from build123d import *

# Parameters (mm, degrees)
EXTRUDE_1_DEPTH = 10
FILLET_1_R      = 1


with BuildPart() as part:
    # 草图4 → 凸台-拉伸1 (new body)
    with BuildSketch(Plane.XY):
        Polygon((-29, 35), (-35, 35), (-35, 2), (-29, 2), (-29, -20), (-35, -20), (-35, -35), (35, -35), (35, 35), (29, 35), (29, 34), (17, 34), (17, 35), (-17, 35), (-17, 34), (-29, 34), align=None)
    extrude(amount=EXTRUDE_1_DEPTH)

    # 圆角1
    fillet_1_edges = [part.edges().sort_by_distance(p)[0] for p in [
        (-29, -20, 5),
        (-29, 2, 5),
        (29, 34, 5),
        (17, 34, 5),
        (-17, 34, 5),
        (-29, 34, 5),
    ]]
    fillet(fillet_1_edges, radius=FILLET_1_R - 0.0001)  # a hair under: the kernel refuses the full size


solid = part.part
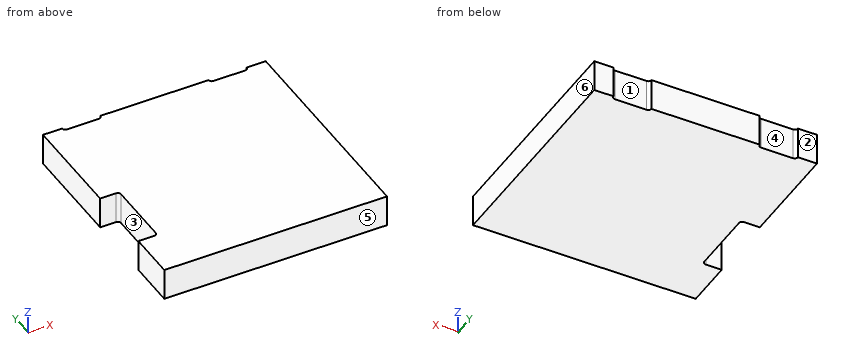
Verification items for the finished model (mm, model axes). Face numbers are marked on the shaded views. A direction names the side the tool comes from. Coordinates: 2 decimals unless noted, no trailing zeros. Order: outer loops, then holes, each group sorted by start corner. A loop starts at its lowest first (then second) coordinate and runs counter-clockwise, first axis right, second up. Notation, with made-up numbers: (-21, 6) -> (38, 6) arc R23 cw to (38, 21) -> close; hole circle Ø3 at (-2.75, 68.25). An arc over 180 degrees is marked (long way). Use CSV: the item, a comma, the result in double quotes. Start each with the question number.
Q1. Tool access check on the marked faces 1, 2 and 3. Record the directions out of +Z, -Z, +X, -X, +Y, -Y that give a thin tool (end or side, any length) a straight path to the whole face; none if there is none.
Q2. Section check B-B, the plane y = -7. Record the cut outline in (x, z).
Q3. Draft check along X on the marked faces 4, 5 and 6. Enter one of: +X half, -X half, draft (parallel to the pull), parting line (faces both ways), or undercut.
Q4. Thickness scan on line 1 along Y through (x, z) = (-31.5, 4.5); line 2 along X through (y, z) = (-11, 8.75); line 3 along Y through (x, z) = (-22, 2.5). Record the ranges inside material, lowest first.
Returned:
1,face 1,"+Z, -Z, +Y"
1,face 2,"+Z, -Z, +X, -X, +Y"
1,face 3,"+Z, -Z, -X"
2,outline,"(-29, 0) -> (35, 0) -> (35, 10) -> (-29, 10) -> close"
3,face 4,"undercut"
3,face 5,"draft"
3,face 6,"+X half"
4,line 1,"y = -35 to -20, 2 to 35"
4,line 2,"x = -29 to 35"
4,line 3,"y = -35 to 34"
